from build123d import *

# Parameters (mm, degrees)
SKETCH1_W           = 57.667844522
SKETCH1_H           = 30
BOSS_EXTRUDE1_DEPTH = 30
SKETCH2_R           = 4
CUT_EXTRUDE2_DEPTH  = 40
SKETCH4_R           = 8
SKETCH4_R_2         = 4
CUT_EXTRUDE3_DEPTH  = 31
SKETCH5_R           = 3
CUT_EXTRUDE4_DEPTH  = 4
SKETCH6_R           = 9.45
CUT_EXTRUDE6_DEPTH  = 31
BOSS_EXTRUDE2_DEPTH = 30
SKETCH8_W           = 0.5
SKETCH8_H           = 6.199937256
CUT_EXTRUDE7_DEPTH  = 31


with BuildPart() as part:
    # Sketch1 → Boss-Extrude1 (new body)
    with BuildSketch(Plane(origin=(0, 0, 0), x_dir=(1, 0, 0), z_dir=(0, 1, 0))):
        Rectangle(SKETCH1_W, SKETCH1_H)
    extrude(amount=BOSS_EXTRUDE1_DEPTH)

    # Sketch2 → Cut-Extrude2 (cut)
    with BuildSketch(Plane(origin=(0, 30, 0), x_dir=(1, 0, 0), z_dir=(0, 1, 0))):
        with Locations((0, 4)):
            Circle(SKETCH2_R)
    extrude(amount=-CUT_EXTRUDE2_DEPTH, mode=Mode.SUBTRACT)

    # Sketch4 → Cut-Extrude3 (cut, through all)
    with BuildSketch(Plane(origin=(0, 30, 0), x_dir=(1, 0, 0), z_dir=(0, 1, 0))):
        with Locations((0, 4)):
            Circle(SKETCH4_R)
        with Locations((0, 4)):
            Circle(SKETCH4_R_2, mode=Mode.SUBTRACT)
        with BuildLine():
            ThreePointArc((-11, 4), (-7.778174609, 11.778174577), (-4.5e-08, 15))
            Line((-4.5e-08, 15), (-28.833922261, 15))
            Line((-28.833922261, 15), (-28.833922261, -12))
            Line((-28.833922261, -12), (-11, -12))
            Line((-11, -12), (-11, 4))
        make_face()
        with BuildLine():
            ThreePointArc((-4.5e-08, 15), (7.778174577, 11.778174609), (11, 4))
            Line((11, 4), (11, -12))
            Line((11, -12), (28.833922261, -12))
            Line((28.833922261, -12), (28.833922261, 15))
            Line((28.833922261, 15), (-4.5e-08, 15))
        make_face()
        with BuildLine():
            Line((7.549834435, -12), (7.549834435, -4))
            ThreePointArc((7.549834435, -4), (0, -7), (-7.549834435, -4))
            Line((-7.549834435, -4), (-7.549834435, -12))
            Line((-7.549834435, -12), (7.549834435, -12))
        make_face()
    extrude(amount=-CUT_EXTRUDE3_DEPTH, mode=Mode.SUBTRACT)

    # Sketch5 → Cut-Extrude4 (cut, through all)
    with BuildSketch(Plane(origin=(0, 0, 12), x_dir=(-1, 0, 0), z_dir=(0, 0, -1))):
        with Locations((-19.916961131, 23)):
            Circle(SKETCH5_R)
        with Locations((19.916961131, 23)):
            Circle(SKETCH5_R)
    extrude(amount=-CUT_EXTRUDE4_DEPTH, mode=Mode.SUBTRACT)

    # Sketch6 → Cut-Extrude6 (cut, through all)
    with BuildSketch(Plane(origin=(0, 30, 0), x_dir=(1, 0, 0), z_dir=(0, 1, 0))):
        with Locations((0, 4)):
            Circle(SKETCH6_R)
    extrude(amount=-CUT_EXTRUDE6_DEPTH, mode=Mode.SUBTRACT)

    # Sketch7 → Boss-Extrude2 (add, through all)
    with BuildSketch(Plane(origin=(0, 30, 0), x_dir=(1, 0, 0), z_dir=(0, 1, 0))):
        with BuildLine():
            Line((11, 4), (11, -12))
            Line((11, -12), (12.001946675, -12))
            Line((12.001946675, -12), (12.001946675, 4))
            ThreePointArc((12.001946675, 4), (0, 16.001946675), (-12.001946675, 4))
            Line((-12.001946675, 4), (-12.001946675, -12))
            Line((-12.001946675, -12), (-11, -12))
            Line((-11, -12), (-11, 4))
            ThreePointArc((-11, 4), (0, 15), (11, 4))
        make_face()
        with BuildLine():
            ThreePointArc((-7.549834435, -5.329883385), (0, -8.001946675), (7.549834435, -5.329883385))
            Line((7.549834435, -5.329883385), (7.549834435, -4))
            ThreePointArc((7.549834435, -4), (0, -7), (-7.549834435, -4))
            Line((-7.549834435, -4), (-7.549834435, -5.329883385))
        make_face()
    extrude(amount=-BOSS_EXTRUDE2_DEPTH)

    # Sketch8 → Cut-Extrude7 (cut, through all)
    with BuildSketch(Plane(origin=(0, 30, 0), x_dir=(1, 0, 0), z_dir=(0, 1, 0))):
        with Locations((0.121996235, 15.101825576)):
            Rectangle(SKETCH8_W, SKETCH8_H)
    extrude(amount=-CUT_EXTRUDE7_DEPTH, mode=Mode.SUBTRACT)


solid = part.part
Can you work these out from the model? Positions are in its coordinate system, mm. A direction names the side the tool comes from. Coordinates: 2 decimals unless noted, no trailing zeros. Write each loop counter-clockwise with the first axis right and the second up, starting at its lowest first coordinate (ties: lowest second). Pieces come first, ordered by that corner, then holes. Notation, with made-up numbers: (14.25, -8) -> (43.25, -8) arc R23 ccw to (43.25, 20) -> close; hole circle Ø8 at (-2, -26). An arc over 180 degrees is marked (long way). Answer as CSV lines item,"result".
1) If I drill on line 1 (Z direction, x = 0, y = 7.75); line 2 (X direction, y = 2, z = 10.5); line 3 (Z direction, x = 5.5, y = 16.5), over which ranges is the centre line in solid material (lowest first)? Write a range as from..to.
Check result:
line 1,"5.45..8, 12..15"
line 2,"-12..-7.55, 7.55..12"
line 3,"-14.67..-11.68, 3.68..6.67, 12..15"
2) If we mould it in two halves opening along Z, with no side actions, what happens to faces 1 (the flat face through (0, 15, 12)), 2 (the flat face through (0, 15, 15)), 3 (the flat face through (0.372, 15, -15)), 4 (the flat face through (-21, 15, 12))? For each: +Z half, -Z half, draft (parallel to the pull), parting line (faces both ways), or undercut.
Check result:
face 1,"undercut"
face 2,"+Z half"
face 3,"draft"
face 4,"-Z half"
3) If we section it at D-D on y = 8.5: Please give me the cut outline in (x, z), then the cut area to 3 significant figures.
Check result:
outline,"(-28.83, 12) -> (-12, 12) -> (-12, -4) arc R12 ccw to (-0.13, -16) -> (-0.13, -13.45) arc R9.45 cw (long way) to (0.37, -13.44) -> (0.37, -16) arc R12 ccw to (12, -4) -> (12, 12) -> (28.83, 12) -> (28.83, 15) -> (-28.83, 15) -> close; hole (-7.55, 5.33) arc R12 cw to (7.55, 5.33) -> (7.55, 12) -> (-7.55, 12) -> close"
area,"428 mm²"
4) If we section it at C-C on x = -22: Please give me the cut outline in (y, z), then the cut area to 3 significant figures.
Check result:
outline,"(0, 12) -> (20.84, 12) -> (20.84, 15) -> (0, 15) -> close; (25.16, 12) -> (30, 12) -> (30, 15) -> (25.16, 15) -> close"
area,"77.0 mm²"
5) Will these pins go through, and if not, where does the flat tip stop? P1, Ø4, axis at y = 22.5, z = -12.5, coming from the +X side; P2, Ø1.5, axis at y = 9, z = 0, coming from the +X side; P3, Ø12, axis at x = 19.5, z = -4.5, coming from the -Y side; P4, Ø5, axis at x = 22.5, y = 11.5, coming from the -Z side.
Check result:
P1,"x = 10.09"
P2,"x = 12"
P3,"through"
P4,"z = 12"
6) If we section it at B-B on z = 9: Please give me the cut outline in (x, y).
Check result:
outline,"(-12, 0) -> (-7.55, 0) -> (-7.55, 30) -> (-12, 30) -> close; (7.55, 0) -> (12, 0) -> (12, 30) -> (7.55, 30) -> close"
7) If we section it at A-A on y = 24.25: Please give me the cut outline in (x, z), then the cut area to 3 significant figures.
Check result:
outline,"(-28.83, 12) -> (-22.64, 12) -> (-22.64, 15) -> (-28.83, 15) -> close; (-17.19, 12) -> (-12, 12) -> (-12, -4) arc R12 ccw to (-0.13, -16) -> (-0.13, -13.45) arc R9.45 cw (long way) to (0.37, -13.44) -> (0.37, -16) arc R12 ccw to (12, -4) -> (12, 12) -> (17.19, 12) -> (17.19, 15) -> (-17.19, 15) -> close; (22.64, 12) -> (28.83, 12) -> (28.83, 15) -> (22.64, 15) -> close; hole (-7.55, 5.33) arc R12 cw to (7.55, 5.33) -> (7.55, 12) -> (-7.55, 12) -> close"
area,"396 mm²"
8) On a 3-axis mill with a long thin cutter (end or side, diameter ignored), from which of +Z, -Z, +X, -X, +Y, -Y can I reach the whole of each face in a straight line? I mean faces 5 (the flat face through (-0.128, 15, -15)), 6 (the flat face through (-12.002, 15, 4)), 7 (the flat face through (7.55, 15, 9)), 8 (the flat face through (20, 15, 12)). Say none if no direction works.
Check result:
face 5,"-Z, +Y, -Y"
face 6,"-Z, -X, +Y, -Y"
face 7,"+Y, -Y"
face 8,"-Z, +X, +Y, -Y"
